Model file for the job. Use its own axes, mm. Coordinates: 2 decimals unless noted, no trailing zeros. Write each loop counter-clockwise with the first axis right and the second up, starting at its lowest first coordinate (ties: lowest second). Pieces come first, ordered by that corner, then holes.
Q1. Band-saw the part on A-A, the plane y = 203.2. Write the cut outline in (x, z), plus the area to 3 significant figures.
Q2. Band-saw the part on B-B, the plane x = 203.2. Write the cut outline in (y, z), plus the area to 3 significant figures.
Q3. Drill centre lines: probe 1 along Y at (x, z) = (203.2, 5.75); probe 2 along X at (y, z) = (203.2, 5.5). Where is each one in solid material? Low to high.
Q4. Pull direction Y, two halves, no side cores. Call faces 1 (the flat face through (125, 0, 6)), 2 (the flat face through (254, 150, 6)), 3 (the cylindrical face through (189.034, 205.06, 6.261)): released by +Y, released by -Y, zero draft, split by the parting line, or undercut.
Autodesk Inventor part; units mm, degrees
ref_plane "YZ Plane" through (0, 0, 0) normal (1, 0, 0) x (0, 1, 0)
ref_plane "XZ Plane" through (0, 0, 0) normal (0, 1, 0) x (-1, 0, 0)
ref_plane "XY Plane" through (0, 0, 0) normal (0, 0, 1) x (1, 0, 0)
sketch "Sketch1" plane through (0, 0, 0) normal (0, 0, 1) x (1, 0, 0)
  line L0 (0, 0) -> (254, 0)
  line L1 (254, 0) -> (254, 304.8)
  line L2 (254, 304.8) -> (0, 304.8)
  line L3 (0, 304.8) -> (0, 0)
  dimension "d0" = 254
  dimension "d1" = 304.8
extrude "Extrusion1" add sketch "Sketch1" along normal blind 12.7
sketch "Sketch2" plane through (0, 0, 12.7) normal (0, 0, 1) x (1, 0, 0)
  line L0 (0, 0) -> (254, 0)
  line L1 (254, 0) -> (254, 304.8)
  point P0 (203.2, 203.2)
  dimension "d11" = 203.2
  dimension "d12" = 50.8
hole "Hole1" at (203.2, 203.2, 12.7) direction (0, 0, -1) diameter 28.575 end through all
properties part number "Shaft Mount" material "Wood (Maple)"
Answer sheet:
1. outline: (0, 0) - (188.91, 0) - (188.91, 12.7) - (0, 12.7) - close; (217.49, 0) - (254, 0) - (254, 12.7) - (217.49, 12.7) - close
1. area: 2,860 mm2
2. outline: (0, 0) - (188.91, 0) - (188.91, 12.7) - (0, 12.7) - close; (217.49, 0) - (304.8, 0) - (304.8, 12.7) - (217.49, 12.7) - close
2. area: 3,510 mm2
3. probe 1: y = 0 to 188.91, 217.49 to 304.8
3. probe 2: x = 0 to 188.91, 217.49 to 254
4. face 1: released by -Y
4. face 2: zero draft
4. face 3: undercut
